from build123d import *

# Parameters (mm, degrees)
BOSS_EXTRUDE1_DEPTH = 187
CUT_EXTRUDE3_DEPTH  = 135
SKETCH3_W           = 208.90375788
SKETCH3_H           = 100
CUT_EXTRUDE4_DEPTH  = 175
SKETCH4_R           = 45
BOSS_EXTRUDE2_DEPTH = 5
BOSS_EXTRUDE3_START = 5
SKETCH5_R           = 45
BOSS_EXTRUDE3_DEPTH = 5
SKETCH6_W           = 13.051719475
SKETCH6_H           = 51.345683967
BOSS_EXTRUDE4_DEPTH = 5
BOSS_EXTRUDE5_DEPTH = 5
SKETCH8_R           = 15.225
CUT_EXTRUDE6_DEPTH  = 2


with BuildPart() as part:
    # Sketch1 → Boss-Extrude1 (new body)
    with BuildSketch(Plane(origin=(0, 0, 0), x_dir=(1, 0, 0), z_dir=(0, 1, 0))):
        with BuildLine():
            Line((0, 70), (-251.769125683, 75))
            Line((-251.769125683, 75), (-251.769125683, -75))
            Line((-251.769125683, -75), (0, -70))
            ThreePointArc((0, -70), (70, 0), (0, 70))
        make_face()
    extrude(amount=-BOSS_EXTRUDE1_DEPTH)

    # Sketch2 → Cut-Extrude3 (cut)
    with BuildSketch(Plane(origin=(1.38961445, 0, 69.972403001), x_dir=(0.9998028591480678, 0, -0.019855549333850253), z_dir=(0.019855549333850253, 0, 0.9998028591480679))):
        Polygon((-1.389888453, -43.5), (169.277022147, -43.5), (169.277022147, -143.5), (-1.389888453, -143.5), (-65.389888453, -143.5), (-65.389888453, -43.5), align=None)
    extrude(amount=-CUT_EXTRUDE3_DEPTH, mode=Mode.SUBTRACT)

    # Sketch3 → Cut-Extrude4 (cut)
    with BuildSketch(Plane(origin=(-1.29088471, 0, -65.000982984), x_dir=(0.9998028591480678, 0, -0.019855549333850163), z_dir=(0.019855549333850163, 0, 0.9998028591480679))):
        with Locations((39.061990487, -93.5)):
            Rectangle(SKETCH3_W, SKETCH3_H)
    extrude(amount=CUT_EXTRUDE4_DEPTH, mode=Mode.SUBTRACT)

    # Sketch4 → Boss-Extrude2 (add)
    with BuildSketch(Plane(origin=(0, 0, 0), x_dir=(1, 0, 0), z_dir=(0, 1, 0))):
        with Locations(Location((0, 0, 0), (0, 0, 270))):
            Circle(SKETCH4_R)
    extrude(amount=BOSS_EXTRUDE2_DEPTH)

    # Sketch5 → Boss-Extrude3 (add)
    with BuildSketch(Plane.XZ.offset(187).offset(BOSS_EXTRUDE3_START)):
        with Locations(Location((0, 0, 0), (0, 0, 90))):
            Circle(SKETCH5_R)
    extrude(amount=-BOSS_EXTRUDE3_DEPTH)

    # Sketch6 → Boss-Extrude4 (add)
    with BuildSketch(Plane(origin=(1.38961445, 0, 69.972403001), x_dir=(0.9998028591480678, 0, -0.019855549333850253), z_dir=(0.019855549333850253, 0, 0.9998028591480679))):
        with Locations((-71.915748191, -92.016210874)):
            Rectangle(SKETCH6_W, SKETCH6_H)
    extrude(amount=BOSS_EXTRUDE4_DEPTH)

    # Sketch7 → Boss-Extrude5 (add)
    with BuildSketch(Plane(origin=(1.38961445, 0, 69.972403001), x_dir=(0.9998028591480678, 0, -0.019855549333850253), z_dir=(0.019855549333850253, 0, 0.9998028591480679))):
        with BuildLine():
            Line((-108.508236533, -116.799531344), (-108.508236533, -69.172508895))
            ThreePointArc((-108.508236533, -69.172508895), (-103.774379298, -64.438651661), (-99.040522064, -69.172508895))
            Line((-99.040522064, -69.172508895), (-99.040522064, -116.799531344))
            ThreePointArc((-99.040522064, -116.799531344), (-103.774379298, -121.533388578), (-108.508236533, -116.799531344))
        make_face()
    extrude(amount=BOSS_EXTRUDE5_DEPTH)

    # Sketch8 → Cut-Extrude6 (cut)
    with BuildSketch(Plane(origin=(0, 0, 0), x_dir=(1, 0, 0), z_dir=(0, 1, 0))):
        with Locations(Location((-229.928260902, 0, 0), (0, 0, 270))):
            Circle(SKETCH8_R)
    extrude(amount=-CUT_EXTRUDE6_DEPTH, mode=Mode.SUBTRACT)


solid = part.part
For this review, take the finished solid that the model builds, in its own axes (mm). A direction names the side the tool comes from. Give positions to 0.01 mm unless a question says otherwise; leave off trailing zeros. Loops run counter-clockwise (first coordinate to the right, second up) from the corner with the lowest first, then second, coordinate; pieces in that order, holes last.
Item 1: Draft analysis for pull direction Y (two halves, no side actions). For faces 3 (the flat face through (-93, 0, -1)), 4 (the flat face through (3, -43.5, 3)), 5 (the flat face through (-129, -187, -1)), 6 (the cylindrical face through (17.235, -189.535, 41.569)), state which applies: +Y half, -Y half, draft (parallel to the pull), parting line (faces both ways), or undercut.
Item 2: Insertion check: pin 1 (4 mm diameter, centred on x = -70, z = 74.5, fed in from -Y); pin 2 (1 mm diameter, centred on y = -116.5, z = -6, fed in from +X); pin 3 (10 mm diameter, centred on x = -175.5, y = -138.5, fed in from -Z). Each pin has a flat end and moves straight along its axis. Give the tip position at first contact, or say it passes through.
Item 3: Tool access review of faces 1 (the flat face through (-1, -192, -1)), 2 (the cylindrical face through (-214.833, -0.986, -1.982)): name each direction out of +Z, -Z, +X, -X, +Y, -Y from which nothing blocks a thin tool from reaching the whole face with its end or side.
Item 4: Take a section at A-A, the plane y = -109. State the section outline as (x, z) points, and give its area (3 significant figures).
Item 5: Take a section at D-D, the plane z = 0. State the section outline as (x, y) points, and give its area (3 significant figures).
Item 6: For line 1 along X through (y, z) = (-1.05, 0); line 2 along Y through (x, z) = (-36, -42); line 3 along Y through (x, z) = (-7.5, 39.5), list the stretches that pass through material, from the lowest coordinate up.
Item 7: Take a section at B-B, the plane z = 57. State the section outline as (x, y) points.
Item 8: Take a section at C-C, the plane x = -40. State the section outline as (y, z) points, and give its area (3 significant figures).
Calculated:
1. face 3: +Y half
1. face 4: undercut
1. face 5: -Y half
1. face 6: draft
2. pin 1: stops at y = -117.69
2. pin 2: stops at x = -65.51
2. pin 3: stops at z = -73.58
3. face 1: +Z, -Z, +X, -X, -Y
3. face 2: +Y
4. outline: (-251.77, -75) - (0, -70) arc R70 ccw to (24.65, -65.52) - (-66.67, -63.7) - (-63.89, 76.27) - (-76.94, 76.53) - (-77.04, 71.53) - (-97.63, 71.94) - (-97.53, 76.94) - (-107, 77.13) - (-107.1, 72.13) - (-251.77, 75) - close
4. area: 27,900 mm2
5. outline: (-251.77, -187) - (-45, -187) - (-45, -192) - (45, -192) - (45, -187) - (70, -187) - (70, -143.5) - (-65.4, -143.5) - (-65.4, -43.5) - (70, -43.5) - (70, 0) - (45, 0) - (45, 5) - (-45, 5) - (-45, 0) - (-214.7, 0) - (-214.7, -2) - (-245.15, -2) - (-245.15, 0) - (-251.77, 0) - close
5. area: 47,500 mm2
6. line 1: x = -251.77 to -245.15, -214.7 to 70
6. line 2: y = -187 to -143.5, -43.5 to 0
6. line 3: y = -192 to -143.5, -43.5 to 5
7. outline: (-251.77, -187) - (40.63, -187) - (40.63, -143.5) - (-64.27, -143.5) - (-64.27, -43.5) - (40.63, -43.5) - (40.63, 0) - (-251.77, 0) - close
8. outline: (-192, -20.62) - (-187, -20.62) - (-187, -70.79) - (0, -70.79) - (0, -20.62) - (5, -20.62) - (5, 20.62) - (0, 20.62) - (0, 70.79) - (-43.5, 70.79) - (-43.5, -64.23) - (-143.5, -64.23) - (-143.5, 70.79) - (-187, 70.79) - (-187, 20.62) - (-192, 20.62) - close
8. area: 13,400 mm2
